Verification items for the finished model (mm, model axes). Face numbers are marked on the shaded views. A direction names the side the tool comes from. Give positions to 0.01 mm unless a question says otherwise; leave off trailing zeros. Order: outer loops, then holes, each group sorted by start corner. A loop starts at its lowest first (then second) coordinate and runs counter-clockwise, first axis right, second up.
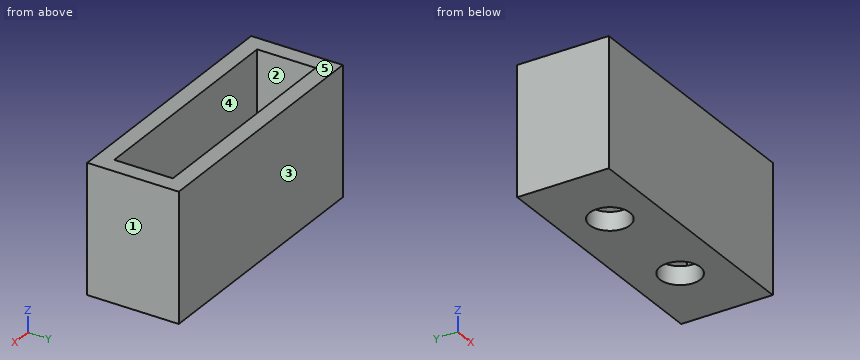
from build123d import *

# Parameters (mm, degrees)
SOFT_CONTACT_AND_WRAP_START     = -1
SOFT_CONTACT_AND_WRAP_PROFILE_W = 14
SOFT_CONTACT_AND_WRAP_PROFILE_H = 5
SOFT_CONTACT_AND_WRAP_DEPTH     = 7
FINGER_SLIP_POCKET_PROFILE_W    = 12.2
FINGER_SLIP_POCKET_PROFILE_H    = 3.2
OPEN_TOP_SLIP_POCKET_DEPTH      = 7
PAD_CAPTURE_M2_START            = -50
PAD_CAPTURE_M2_PROFILE_R        = 1.1
PAD_CAPTURE_M2_DEPTH            = 85.928498393


with BuildPart() as part:
    # Soft_contact_and_wrap_profile → Soft_contact_and_wrap (new body)
    with BuildSketch(Plane.XY.offset(SOFT_CONTACT_AND_WRAP_START)):
        with Locations((21, -17.5)):
            Rectangle(SOFT_CONTACT_AND_WRAP_PROFILE_W, SOFT_CONTACT_AND_WRAP_PROFILE_H)
    extrude(amount=SOFT_CONTACT_AND_WRAP_DEPTH)

    # Finger_slip_pocket_profile → Open_top_slip_pocket (cut)
    with BuildSketch(Plane.XY):
        with Locations((21, -17.5)):
            Rectangle(FINGER_SLIP_POCKET_PROFILE_W, FINGER_SLIP_POCKET_PROFILE_H)
    extrude(amount=OPEN_TOP_SLIP_POCKET_DEPTH, mode=Mode.SUBTRACT)

    # Pad_capture_M2_profile → Pad_capture_M2 (cut, through all)
    with BuildSketch(Plane.XY.offset(PAD_CAPTURE_M2_START)):
        with Locations(Location((18, -17.5, 0), (0, 0, 180))):
            Circle(PAD_CAPTURE_M2_PROFILE_R)
        with Locations(Location((24, -17.5, 0), (0, 0, 180))):
            Circle(PAD_CAPTURE_M2_PROFILE_R)
    extrude(amount=PAD_CAPTURE_M2_DEPTH, mode=Mode.SUBTRACT)


solid = part.part
(1) Section check C-C, the plane z = 4. Enter the section's corners in (x, y), then the cut area to 3 significant figures.
Solved:
outline: (14, -20) - (28, -20) - (28, -15) - (14, -15) - close; hole (14.9, -19.1) - (27.1, -19.1) - (27.1, -15.9) - (14.9, -15.9) - close
area: 31.0 mm2
(2) Scan lines: line 1 (X direction, y = -18.45, z = 2.75); line 2 (Y direction, x = 24, z = -0.75); line 3 (Y direction, x = 19, z = 0.5). Record each from-to range of solid material in increasing order.
Solved:
line 1: x = 14 to 14.9, 27.1 to 28
line 2: y = -20 to -18.6, -16.4 to -15
line 3: y = -20 to -19.1, -15.9 to -15
(3) Go/stop test with flat-tipped pins: pin 1 (2.5 mm diameter, centred on x = 18, y = -17.5, fed in from +Z); pin 2 (1.8 mm diameter, centred on x = 24, y = -17.5, fed in from -Z). Record where each tip stops, or that it passes through.
Solved:
pin 1: stops at z = 0
pin 2: passes through
(4) Set-up check for the marked faces 4 and 5: record each of +Z, -Z, +X, -X, +Y, -Y from which the full face is reachable in a straight line by a thin tool's end or side.
Solved:
face 4: +Z
face 5: +Z, +X, -X, +Y, -Y
(5) Section check A-A, the plane x = 24. Enter the section's corners in (y, z), then the cut area to 3 significant figures.
Solved:
outline: (-20, -1) - (-18.6, -1) - (-18.6, 0) - (-19.1, 0) - (-19.1, 6) - (-20, 6) - close; (-16.4, -1) - (-15, -1) - (-15, 6) - (-15.9, 6) - (-15.9, 0) - (-16.4, 0) - close
area: 13.6 mm2
(6) Release check for a two-part mould opening along Y. For the marked faces 1, 2 and 3 record: pulls with the +Y half, pulls with the -Y half, needs draft (parallel to the pull), parting line crosses it, or undercut.
Solved:
face 1: needs draft
face 2: undercut
face 3: pulls with the +Y half
(7) Section check B-B, the plane y = -17.5. Enter the section's corners in (x, z), then the cut area to 3 significant figures.
Solved:
outline: (14, -1) - (16.9, -1) - (16.9, 0) - (14.9, 0) - (14.9, 6) - (14, 6) - close; (19.1, -1) - (22.9, -1) - (22.9, 0) - (19.1, 0) - close; (25.1, -1) - (28, -1) - (28, 6) - (27.1, 6) - (27.1, 0) - (25.1, 0) - close
area: 20.4 mm2
(8) Section check D-D, the plane x = 26. Enter the section's corners in (y, z).
Solved:
outline: (-20, -1) - (-15, -1) - (-15, 6) - (-15.9, 6) - (-15.9, 0) - (-19.1, 0) - (-19.1, 6) - (-20, 6) - close
